Verification items for the finished model (mm, model axes). Give positions to 0.01 mm unless a question says otherwise; leave off trailing zeros. Order: outer loops, then holes, each group sorted by start corner. A loop starts at its lowest first (then second) coordinate and runs counter-clockwise, first axis right, second up. Notation, with made-up numbers: (30.25, -27.75) -> (38.25, -27.75) arc R19 cw to (38.25, -17.75) -> close; hole circle Ø11 at (44.5, -38). An arc over 180 degrees is marked (long way). Write each question's results on one line, items separated by ' | '. Start each with the question number.
1. Depth check by flat-ended pin: pin 1 Ø3 at (x, z) = (6.5, -765) entering from +Y. Enter the tip coordinate at first touch or a pass-through.
2. Material ranges on L1, parallel to Z at x = 3.75, y = -333; L2, parallel to Y at x = 5, z = -467.5, recorded low to high. Write a range as from..to.
3. Cross-section at B-B, the plane x = 4.5. Enter the section's corners in (y, z).
4. Cross-section at A-A, the plane z = -918. Enter the section's corners in (x, y), then the cut area to 3 significant figures.
5. Cross-section at C-C, the plane y = -340. Enter the section's corners in (x, z), then the cut area to 3 significant figures.
Autodesk Inventor part; units mm, degrees
ref_plane "YZ Plane" through (0, 0, 0) normal (1, 0, 0) x (0, 1, 0)
ref_plane "XZ Plane" through (0, 0, 0) normal (0, 1, 0) x (-1, 0, 0)
ref_plane "XY Plane" through (0, 0, 0) normal (0, 0, 1) x (1, 0, 0)
sketch "Sketch1" plane through (0, 0, 0) normal (1, 0, 0) x (0, 1, 0)
  line L0 (0, 0) -> (-490, 0)
  line L1 (-490, 0) -> (-490, -1138)
  line L2 (-490, -1138) -> (0, -1138)
  line L3 (0, -1138) -> (0, 0)
  line L4 (-480, -1128) -> (-480, -10)
  line L5 (-480, -10) -> (-10, -10)
  line L6 (-10, -10) -> (-10, -1128)
  line L7 (-10, -1128) -> (-480, -1128)
  dimension "d0" = 490
  dimension "portaAltura" = 1138
  dimension "d2" = 10
  dimension "portaLargura" = 470
extrude "Extrusion1" add sketch "Sketch1" along normal blind 10
sketch "Sketch2" plane through (0, -490, 0) normal (0, 0, 1) x (1, 0, 0)
  line L0 (0, 490) -> (0, 0)
  line L1 (0, 0) -> (10, 0)
  line L2 (10, 490) -> (10, 0)
  line L3 (0, 490) -> (10, 490)
  line L4 (0, 0) -> (-3.182, -3.182)
  line L5 (0, 0) -> (4.5, 0) construction
  line L6 (0, 490) -> (0, 0)
  circle A0 centre (-3.182, -3.182) radius 5
  circle A1 centre (-3.182, -3.182) radius 4
  dimension "d5" = 4.5
  dimension "d6" = 135
  dimension "d7" = 1
  dimension "d10" = 10
extrude "Extrusion2" [suppressed]
ref_plane "Work Plane1" through (0, 0, -569) normal (0, 0, 1) x (1, 0, 0)
mirror "Mirror1" [suppressed]
fillet "Fillet1" [suppressed]
ref_plane "Work Plane2" through (0, -490, -1113) normal (0, 0, 1) x (1, 0, 0)
sketch "Sketch3" plane through (0, -490, -1113) normal (0, 0, 1) x (1, 0, 0)
  arc A0 (0, 0.6748) -> (0.6748, 0) centre (-3.182, -3.182) ccw
  circle A1 centre (-3.182, -3.182) radius 4
  line L0 (0.6748, 0) -> (10, 0)
  circle A2 centre (-3.182, -3.182) radius 5
  point P0 (0, 490)
  point P1 (0, 0.6748)
extrude "Extrusion3" [suppressed]
sketch "Sketch4" plane through (0, 0, 0) normal (0, 0, 1) x (1, 0, 0)
  circle A0 centre (-3.182, -493.182) radius 4
  arc A1 (0, -489.3252) -> (0.6748, -490) centre (-3.182, -493.182) ccw
  circle A2 centre (-3.182, -493.182) radius 4
  line L0 (0, -490) -> (10, -490)
  circle A3 centre (-3.182, -493.182) radius 5
  point P0 (0, 0)
  point P1 (0, -489.3252)
extrude "Extrusion4" [suppressed]
sketch "Sketch5" plane through (0, -490, -35) normal (0, 0, -1) x (-1, 0, 0)
  circle A0 centre (3.182, -3.182) radius 4
  arc A1 (-0.6748, 0) -> (0, 0.6748) centre (3.182, -3.182) ccw
  circle A2 centre (3.182, -3.182) radius 5
  point P0 (0, 490)
  point P1 (0, 0.6748)
extrude "Extrusion5" [suppressed]
sketch "Sketch6" plane through (0, 0, 0) normal (0, 0, 1) x (1, 0, 0)
  line L0 (0, -490) -> (10, -490)
  line L1 (10, 0) -> (10, -490)
  line L2 (0, 0) -> (10, 0)
  line L3 (0, 0) -> (0, -490)
  line L4 (10, -490) -> (10, 0) construction
  line L5 (0, -10) -> (10, -10) construction
  line L6 (10, 0) -> (0, -10) construction
  line L7 (0, 0) -> (10, 0) construction
  line L8 (0, 0) -> (10, -10) construction
  circle A0 centre (5, -5) radius 2.5
  dimension "d19" = 5
extrude "Extrusion6" [suppressed]
sketch "Sketch7" plane through (5, -5, 10) normal (0, 0, 1) x (1, 0, 0)
  circle A0 centre (0, 0) radius 2.5
  circle A1 centre (0, 0) radius 5
  point P0 (-5, 5)
  dimension "d22" = 10
extrude "Extrusion7" [suppressed]
mirror "Mirror2" [suppressed]
properties part number "porta1"
Results below:
1) pin 1: stops at y = 0
2) L1: z = -1138..-1128, -10..0 | L2: y = -490..-480, -10..0
3) outline: (-490, -1138) -> (0, -1138) -> (0, 0) -> (-490, 0) -> close; hole (-480, -1128) -> (-10, -1128) -> (-10, -10) -> (-480, -10) -> close
4) outline: (0, -490) -> (10, -490) -> (10, -480) -> (0, -480) -> close; (0, -10) -> (10, -10) -> (10, 0) -> (0, 0) -> close | area: 200 mm²
5) outline: (0, -1138) -> (10, -1138) -> (10, -1128) -> (0, -1128) -> close; (0, -10) -> (10, -10) -> (10, 0) -> (0, 0) -> close | area: 200 mm²
